CAD build for the part. Positions are in the model's coordinates, mm. A direction names the side the tool comes from. Give positions to 0.01 mm unless a question says otherwise; leave off trailing zeros. Order: outer loops, then holes, each group sorted by start corner. A loop starts at its lowest first (then second) coordinate and runs counter-clockwise, first axis right, second up.
Item 1: Flat gauge pins, fed straight in: P1, Ø1.5, axis at y = 17, z = -11, coming from the -X side; P2, Ø10, axis at x = 1, z = -16.5, coming from the +Y side; P3, Ø4, axis at x = 6, z = 4, coming from the +Y side; P4, Ø6, axis at x = 12, z = 5, coming from the -Y side. Where does each tip first touch, or does it go through?
Item 2: Band-saw the part on C-C on y = 23.75. Give the cut face in (x, z).
Item 3: Band-saw the part on B-B on z = 3.5. Give the cut face in (x, y), plus the area to 3 significant figures.
Item 4: Band-saw the part on A-A on y = 19.5. Give the cut face in (x, z) (3 decimals).
Item 5: Wall check: L1, parallel to X at y = 22.75, z = -18; L2, parallel to X at y = 1.75, z = -2.5; L3, parallel to Z at x = 1.5, y = 11.25. Give the ranges that are in metal, low to high.
Item 6: Which spindle directions (+Z, -Z, +X, -X, +Y, -Y) get a long thin tool onto all of the face, cutting with end or side? Do faces 1 (the flat face through (8.89, 25, -10)), 2 (the cylindrical face through (17.83, 8.38, -11.75)), 3 (the flat face through (7, 25, 0)), 4 (the flat face through (18, 10, -6.985)). Say none if no direction does.
```python
from build123d import *

# Parameters (mm, degrees)
F0_W      = 20.32
F0_H      = 19.05
F1_DEPTH  = 13.97
F3_START  = -6.985
F2_W      = 29.21
F2_H      = 4.318
F3_DEPTH  = 5.1308
F7_W      = 20.32
F7_H      = 9.525
F8_DEPTH  = 1.905
F9_DEPTH  = 9.525
F10_R     = 1.27
F12_DEPTH = 25.4


with BuildPart() as f1:
    # F0 (on Right) → F1 (new body)
    with BuildSketch(Plane.YZ):
        with Locations((10.16, -9.525)):
            Rectangle(F0_W, F0_H)
    extrude(amount=F1_DEPTH)

    # F2 (on face) → F3 (join)
    with BuildSketch(Plane.XY.offset(F3_START)):
        with Locations((6.985, 10.16)):
            Rectangle(F2_W, F2_H)
    extrude(amount=-F3_DEPTH)

    # F5 (on offset) → F6 (revolve)
    with BuildSketch(Plane.YZ.offset(6.985)):
        Polygon((10.16, -19.05), (5.715, -19.05), (10.16, -25.4), align=None)
    revolve(axis=Axis((6.985, 10.16, -22.225), (0, 0, 1)))

    # F7 (on offset) → F8 (join, symmetric)
    with BuildSketch(Plane.YZ.offset(6.985)):
        with BuildLine():
            ThreePointArc((20.32, -19.05), (27.0551920908, -16.2601920908), (29.845, -9.525))
            Line((29.845, -9.525), (20.32, -9.525))
            Line((20.32, -9.525), (20.32, -19.05))
        make_face()
        with Locations((10.16, 4.7625)):
            Rectangle(F7_W, F7_H)
    extrude(amount=F8_DEPTH, both=True)

    # F9 (add, through all): a face of the model
    f9_faces = [f1.faces().sort_by_distance(p)[0] for p in [
        (6.985, 25.0825, -9.525),
    ]]
    extrude(f9_faces, amount=F9_DEPTH)

    # F10
    f10_edges = [f1.edges().sort_by_distance(p)[0] for p in [
        (17.78, 8.001, -12.1158),
        (17.78, 12.319, -6.985),
        (-3.81, 8.001, -12.1158),
        (-3.81, 12.319, -6.985),
    ]]
    fillet(f10_edges, radius=F10_R)

    # F11 (on offset) → F12 (cut, symmetric)
    with BuildSketch(Plane.YZ.offset(6.985)):
        Polygon((29.845, -10.16), (29.845, -8.89), (28.1003518386, -9.525), align=None)
    extrude(amount=F12_DEPTH, both=True, mode=Mode.SUBTRACT)


solid = f1.part
```
The answers:
1. P1: stops at x = 0
1. P2: stops at y = 28.92
1. P3: stops at y = 20.32
1. P4: passes through
2. outline: (5.08, -18.41) - (8.89, -18.41) - (8.89, 0) - (5.08, 0) - close
3. outline: (5.08, 0) - (8.89, 0) - (8.89, 20.32) - (5.08, 20.32) - close
3. area: 77.4 mm2
4. outline: (0, -19.05) - (13.97, -19.05) - (13.97, 0) - (8.89, 0) - (8.89, 9.525) - (5.08, 9.525) - (5.08, 0) - (0, 0) - close
5. L1: x = 5.08 to 8.89
5. L2: x = 0 to 13.97
5. L3: z = -19.05 to 0
6. face 1: +Z, -Z, +X, +Y
6. face 2: -Z, +X, -Y
6. face 3: +Z, +X, -X, +Y
6. face 4: +Z, +X, +Y, -Y
